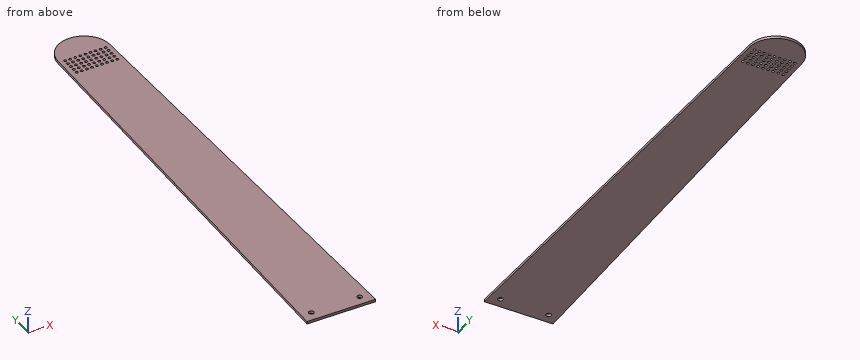
Autodesk Inventor part; units mm, degrees
ref_plane "YZ Plane" through (0, 0, 0) normal (1, 0, 0) x (0, 1, 0)
ref_plane "XZ Plane" through (0, 0, 0) normal (0, 1, 0) x (-1, 0, 0)
ref_plane "XY Plane" through (0, 0, 0) normal (0, 0, 1) x (1, 0, 0)
ref_plane "Work Plane1" through (0, 0, 0) normal (0, 0, 1) x (1, 0, 0)
sketch "Sketch1" plane through (0, 0, 0) normal (0, 0, 1) x (1, 0, 0)
  circle A0 centre (15.2714, 289.6793) radius 1.651
  circle A1 centre (2.5714, 289.6793) radius 1.651
  circle A2 centre (-10.1286, 289.6793) radius 1.651
  circle A3 centre (15.2714, 283.3293) radius 1.651
  circle A4 centre (2.5714, 283.3293) radius 1.651
  circle A5 centre (-10.1286, 283.3293) radius 1.651
  circle A6 centre (15.2714, 276.9793) radius 1.651
  circle A7 centre (2.5714, 276.9793) radius 1.651
  circle A8 centre (-10.1286, 276.9793) radius 1.651
  circle A9 centre (15.2714, 270.6293) radius 1.651
  circle A10 centre (2.5714, 270.6293) radius 1.651
  circle A11 centre (-10.1286, 270.6293) radius 1.651
  circle A12 centre (15.2714, 264.2793) radius 1.651
  circle A13 centre (2.5714, 264.2793) radius 1.651
  circle A14 centre (-10.1286, 264.2793) radius 1.651
  circle A15 centre (-16.4786, 264.2793) radius 1.651
  circle A16 centre (-3.7786, 264.2793) radius 1.651
  circle A17 centre (8.9214, 264.2793) radius 1.651
  circle A18 centre (-16.4786, 270.6293) radius 1.651
  circle A19 centre (-3.7786, 270.6293) radius 1.651
  circle A20 centre (8.9214, 270.6293) radius 1.651
  circle A21 centre (-16.4786, 276.9793) radius 1.651
  circle A22 centre (-3.7786, 276.9793) radius 1.651
  circle A23 centre (8.9214, 276.9793) radius 1.651
  circle A24 centre (-16.4786, 283.3293) radius 1.651
  circle A25 centre (-3.7786, 283.3293) radius 1.651
  circle A26 centre (8.9214, 283.3293) radius 1.651
  circle A27 centre (-16.4786, 289.6793) radius 1.651
  circle A28 centre (-3.7786, 289.6793) radius 1.651
  circle A29 centre (8.9214, 289.6793) radius 1.651
  circle A30 centre (25.4672, -253.1178) radius 1.651
  circle A31 centre (19.1172, -253.1178) radius 1.651
  circle A32 centre (12.7672, -253.1178) radius 1.651
  circle A33 centre (6.4172, -253.1178) radius 1.651
  circle A34 centre (0.0672, -253.1178) radius 1.651
  circle A35 centre (-6.2828, -253.1178) radius 1.651
  circle A36 centre (-12.6328, -253.1178) radius 1.651
  circle A37 centre (-18.9828, -253.1178) radius 1.651
  circle A38 centre (-25.3328, -253.1178) radius 1.651
  circle A39 centre (25.4672, -259.4678) radius 1.651
  circle A40 centre (19.1172, -259.4678) radius 1.651
  circle A41 centre (12.7672, -259.4678) radius 1.651
  circle A42 centre (6.4172, -259.4678) radius 1.651
  circle A43 centre (0.0672, -259.4678) radius 1.651
  circle A44 centre (-6.2828, -259.4678) radius 1.651
  circle A45 centre (-12.6328, -259.4678) radius 1.651
  circle A46 centre (-18.9828, -259.4678) radius 1.651
  circle A47 centre (-25.3328, -259.4678) radius 1.651
  circle A48 centre (25.4672, -265.8178) radius 1.651
  circle A49 centre (19.1172, -265.8178) radius 1.651
  circle A50 centre (12.7672, -265.8178) radius 1.651
  circle A51 centre (6.4172, -265.8178) radius 1.651
  circle A52 centre (0.0672, -265.8178) radius 1.651
  circle A53 centre (-6.2828, -265.8178) radius 1.651
  circle A54 centre (-12.6328, -265.8178) radius 1.651
  circle A55 centre (-18.9828, -265.8178) radius 1.651
  circle A56 centre (-25.3328, -265.8178) radius 1.651
  circle A57 centre (25.4672, -272.1678) radius 1.651
  circle A58 centre (19.1172, -272.1678) radius 1.651
  circle A59 centre (12.7672, -272.1678) radius 1.651
  circle A60 centre (6.4172, -272.1678) radius 1.651
  circle A61 centre (0.0672, -272.1678) radius 1.651
  circle A62 centre (-6.2828, -272.1678) radius 1.651
  circle A63 centre (-12.6328, -272.1678) radius 1.651
  circle A64 centre (-18.9828, -272.1678) radius 1.651
  circle A65 centre (-25.3328, -272.1678) radius 1.651
  circle A66 centre (25.4672, -278.5178) radius 1.651
  circle A67 centre (19.1172, -278.5178) radius 1.651
  circle A68 centre (12.7672, -278.5178) radius 1.651
  circle A69 centre (6.4172, -278.5178) radius 1.651
  circle A70 centre (0.0672, -278.5178) radius 1.651
  circle A71 centre (-6.2828, -278.5178) radius 1.651
  circle A72 centre (-12.6328, -278.5178) radius 1.651
  circle A73 centre (-18.9828, -278.5178) radius 1.651
  circle A74 centre (-25.3328, -278.5178) radius 1.651
  arc A75 (22.3491, 290.0954) -> (-22.3491, 290.0954) centre (0, 289.6793) ccw
  line L0 (-22.3491, 290.0954) -> (-33.0532, -284.8678)
  line L1 (-33.0532, -284.8678) -> (33.0532, -284.8678)
  line L2 (33.0532, -284.8678) -> (22.3491, 290.0954)
  arc A76 (32.4033, -249.9589) -> (-32.4033, -249.9589) centre (0, -250.5622) ccw
  line L3 (-32.4033, -249.9589) -> (-42.9236, -815.0533)
  line L4 (-42.9236, -815.0533) -> (42.9236, -815.0533)
  line L5 (42.9236, -815.0533) -> (32.4033, -249.9589)
  line L6 (-32.4033, -218.1533) -> (33.9104, -218.1533) construction
  point P0 (0, 0)
  dimension "d0" = 596.9
extrude "Extrusion1" add sketch "Sketch1" along normal blind 3.175 contours L2 L1 L0 A76 | L5 L4 L3 L1
sketch "Sketch2" plane through (0, 0, 3.175) normal (0, 0, 1) x (1, 0, 0)
  line L0 (-42.9236, -815.0533) -> (42.9236, -815.0533)
  circle A0 centre (-30.2236, -802.3533) radius 3.175
  line L1 (0, -815.0533) -> (0, -733.814) construction
  circle A1 centre (30.2236, -802.3533) radius 3.175
  point P0 (0, 0)
  dimension "d4" = 6.35
  dimension "d5" = 12.7
  dimension "d6" = 12.7
extrude "Extrusion2" cut sketch "Sketch2" against normal through all
properties part number "octoBotoStemSectD_v01"
Source: CAD feature listing. Evaluate the final solid. Frame: model axes, mm. Coordinates: 2 decimals unless noted, no trailing zeros. Loops run counter-clockwise (first coordinate to the right, second up) from the corner with the lowest first, then second, coordinate; pieces in that order, holes last. Notation, with made-up numbers: (39, 49) -> (83, 49) arc R22 ccw to (83, 83) -> close; hole circle Ø10 at (-21.5, -32.75). An arc over 180 degrees is marked (long way). Answer in a Markdown table with one row per item. Add a question column.
Q1. Section A-A on z = 0.6. Give the number of separate pieces and of enclosed holes in the cut face, and give its area (3 significant figures).
Q2. Contact query for flat-ended pins moving along their axis: pin 1 Ø1.5 at (y, z) = (-344.5, 1.5) entering from -X; pin 2 Ø1 at (y, z) = (-517.5, 1.5) entering from +X; pin 3 Ø1 at (y, z) = (-288.5, 1.5) entering from -X. Output: stop coordinate, or through.
Q3. Ray query, line 1 along Y through (x, z) = (12.5, 3.05); line 2 along Y through (x, z) = (-19, 2.2); line 3 along Y through (x, z) = (-27.5, 2.75). Return the intervals inside material, ascending.
Q4. Section B-B on y = -538. Return the cut outline in (x, z) (3 decimals).
Computed values:
| question | item | result |
|---|---|---|
| 1 | separate pieces | 1 |
| 1 | enclosed holes | 47 |
| 1 | area | 43,700 mm^2 |
| 2 | pin 1 | stops at x = -34.18 |
| 2 | pin 2 | stops at x = 37.39 |
| 2 | pin 3 | stops at x = -33.13 |
| 3 | line 1 | y = -815.05 to -280.15, -276.89 to -273.8, -270.54 to -267.45, -264.19 to -261.1, -257.84 to -254.75, -251.49 to -220.66 |
| 3 | line 2 | y = -815.05 to -280.17, -276.87 to -273.82, -270.52 to -267.47, -264.17 to -261.12, -257.82 to -254.77, -251.47 to -224.31 |
| 3 | line 3 | y = -815.05 to -803.99, -800.72 to -233.41 |
| 4 | outline | (-37.766, 0) -> (37.766, 0) -> (37.766, 3.175) -> (-37.766, 3.175) -> close |
